Autodesk Inventor part; units mm, degrees
ref_plane "lockwasher_XY" through (0, 0, 0.254) normal (0, 0, 1) x (1, 0, 0)
ref_plane "lockwasher_YZ" through (0, 0, 0.254) normal (1, 0, 0) x (0, 1, 0)
ref_plane "lockwasher_ZX" through (0, 0, 0.254) normal (0, 1, 0) x (0, 0, 1)
sketch "Sketch_2" plane through (0, 0, 0) normal (0, 0, 1) x (1, 0, 0)
  circle A0 centre (0, 0) radius 5.1054
  line L0 (-3.81, 0) -> (-3.2004, 0)
  arc A1 (-3.2004, 0) -> (-3.0074, -1.0946) centre (0, 0) ccw
  line L1 (-3.0074, -1.0946) -> (-3.5802, -1.3031)
  arc A2 (-3.5802, -1.3031) -> (-2.9186, -2.449) centre (0, 0) ccw
  line L2 (-2.9186, -2.449) -> (-2.4516, -2.0572)
  arc A3 (-2.4516, -2.0572) -> (-1.6002, -2.7716) centre (0, 0) ccw
  line L3 (-1.6002, -2.7716) -> (-1.905, -3.2996)
  arc A4 (-1.905, -3.2996) -> (-0.6616, -3.7521) centre (0, 0) ccw
  line L4 (-0.6616, -3.7521) -> (-0.5557, -3.1518)
  arc A5 (-0.5557, -3.1518) -> (0.5557, -3.1518) centre (0, 0) ccw
  line L5 (0.5557, -3.1518) -> (0.6616, -3.7521)
  arc A6 (0.6616, -3.7521) -> (1.905, -3.2996) centre (0, 0) ccw
  line L6 (1.905, -3.2996) -> (1.6002, -2.7716)
  arc A7 (1.6002, -2.7716) -> (2.4516, -2.0572) centre (0, 0) ccw
  line L7 (2.4516, -2.0572) -> (2.9186, -2.449)
  arc A8 (2.9186, -2.449) -> (3.5802, -1.3031) centre (0, 0) ccw
  line L8 (3.5802, -1.3031) -> (3.0074, -1.0946)
  arc A9 (3.0074, -1.0946) -> (3.2004, 0) centre (0, 0) ccw
  line L9 (3.2004, 0) -> (3.81, 0)
  arc A10 (3.81, 0) -> (3.5802, 1.3031) centre (0, 0) ccw
  line L10 (3.5802, 1.3031) -> (3.0074, 1.0946)
  arc A11 (3.0074, 1.0946) -> (2.4516, 2.0572) centre (0, 0) ccw
  line L11 (2.4516, 2.0572) -> (2.9186, 2.449)
  arc A12 (2.9186, 2.449) -> (1.905, 3.2996) centre (0, 0) ccw
  line L12 (1.905, 3.2996) -> (1.6002, 2.7716)
  arc A13 (1.6002, 2.7716) -> (0.5557, 3.1518) centre (0, 0) ccw
  line L13 (0.5557, 3.1518) -> (0.6616, 3.7521)
  arc A14 (0.6616, 3.7521) -> (-0.6616, 3.7521) centre (0, 0) ccw
  line L14 (-0.6616, 3.7521) -> (-0.5557, 3.1518)
  arc A15 (-0.5557, 3.1518) -> (-1.6002, 2.7716) centre (0, 0) ccw
  line L15 (-1.6002, 2.7716) -> (-1.905, 3.2996)
  arc A16 (-1.905, 3.2996) -> (-2.9186, 2.449) centre (0, 0) ccw
  line L16 (-2.9186, 2.449) -> (-2.4516, 2.0572)
  arc A17 (-2.4516, 2.0572) -> (-3.0074, 1.0946) centre (0, 0) ccw
  line L17 (-3.0074, 1.0946) -> (-3.5802, 1.3031)
  arc A18 (-3.5802, 1.3031) -> (-3.81, 0) centre (0, 0) ccw
extrude "Extrusion1" add sketch "Sketch_2" along normal mid plane 0.508
ref_plane "lockwasher_XY" through (0, 0, 0.254) normal (0, 0, 1) x (1, 0, 0)
ref_plane "lockwasher_YZ" through (0, 0, 0.254) normal (1, 0, 0) x (0, 1, 0)
ref_plane "lockwasher_ZX" through (0, 0, 0.254) normal (0, 1, 0) x (0, 0, 1)
properties part number "AT509"
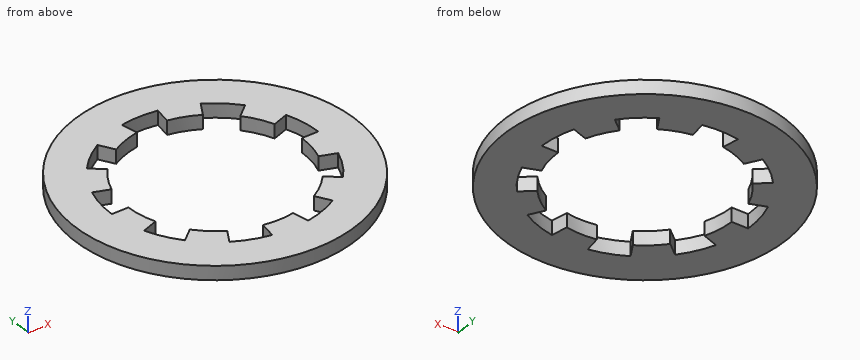
Geometry: final body of the model. Coordinates: model frame, mm. Coordinates: 2 decimals unless noted, no trailing zeros. Order: outer loops, then holes, each group sorted by start corner. A loop starts at its lowest first (then second) coordinate and runs counter-clockwise, first axis right, second up. Notation, with made-up numbers: M 28,88.25 L 66,88.25 A28 ccw 66,121.25 Z; hole C 56.25,-32 d1. An arc over 180 degrees is marked long. Answer in a Markdown table with one row per item. Add a question column.
Q1. Section query B-B on y = 4.5. Return the cut outline in (x, z), and give its area (3 significant figures).
Q2. Contact query for a flat-ended pin moving along its axis: P1, Ø2, axis at x = -1, y = 0, coming from the -Z side. Output: stop coordinate, or through.
Q3. Line query: L1, parallel to X at y = -2.25, z = -0.2; L2, parallel to Y at x = 3.25, z = 0.1; L3, parallel to X at y = 2.25, z = -0.2. Output: solid intervals per line, ascending.
Q4. Section query A-A on x = 0. Return the cut outline in (y, z), and give its area (3 significant figures).
Q5. Section query C-C on x = -4. Return the cut outline in (y, z).
Completed:
| question | item | result |
|---|---|---|
| 1 | outline | M -2.41,-0.25 L 2.41,-0.25 L 2.41,0.25 L -2.41,0.25 Z |
| 1 | area | 2.45 mm2 |
| 2 | P1 | passes through |
| 3 | L1 | x = -4.58 to -3.07, -2.68 to -2.28, 2.28 to 2.68, 3.07 to 4.58 |
| 3 | L2 | y = -3.94 to -1.99, -1.18 to 0, 1.18 to 3.94 |
| 3 | L3 | x = -4.58 to -2.68, 2.68 to 4.58 |
| 4 | outline | M -5.11,-0.25 L -3.2,-0.25 L -3.2,0.25 L -5.11,0.25 Z; M 3.81,-0.25 L 5.11,-0.25 L 5.11,0.25 L 3.81,0.25 Z |
| 4 | area | 1.63 mm2 |
| 5 | outline | M -3.17,-0.25 L 3.17,-0.25 L 3.17,0.25 L -3.17,0.25 Z |
